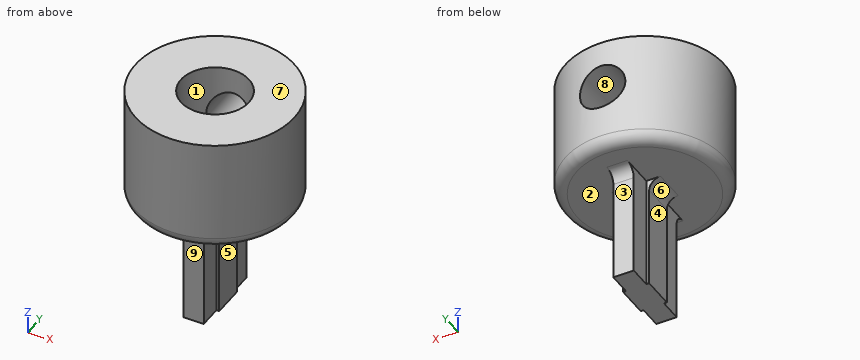
Autodesk Inventor part; units mm, degrees
ref_plane "YZ Plane" through (0, 0, 0) normal (1, 0, 0) x (0, 1, 0)
ref_plane "XZ Plane" through (0, 0, 0) normal (0, 1, 0) x (-1, 0, 0)
ref_plane "XY Plane" through (0, 0, 0) normal (0, 0, 1) x (1, 0, 0)
sketch "Sketch1" plane through (0, 0, 0) normal (0, 0, 1) x (1, 0, 0)
  line L0 (1.25, -1.5) -> (1, -1.5)
  line L1 (1, -1.5) -> (1, -3.5)
  line L2 (1, -3.5) -> (-1, -3.5)
  line L3 (-1, -3.5) -> (-1, -1.5)
  line L4 (-1, -1.5) -> (-1.25, -1.5)
  line L5 (-1.25, -1.5) -> (-1.25, 1.5)
  line L6 (-1.25, 1.5) -> (-1, 1.5)
  line L7 (-1, 1.5) -> (-1, 3.5)
  line L8 (-1, 3.5) -> (1, 3.5)
  line L9 (1, 3.5) -> (1, 1.5)
  line L10 (1, 1.5) -> (1.25, 1.5)
  line L11 (1.25, 1.5) -> (1.25, -1.5)
  circle A0 centre (4.5, 0) radius 1.55
  circle A1 centre (-4.5, 0) radius 1.55
  circle A2 centre (0, 0) radius 8
  line L12 (-0.9, -1.4) -> (-0.9, -3.4)
  line L13 (-0.9, -3.4) -> (0.9, -3.4)
  line L14 (0.9, -3.4) -> (0.9, -1.4)
  line L15 (0.9, -1.4) -> (1.15, -1.4)
  line L16 (1.15, -1.4) -> (1.15, 1.4)
  line L17 (1.15, 1.4) -> (0.9, 1.4)
  line L18 (0.9, 1.4) -> (0.9, 3.4)
  line L19 (0.9, 3.4) -> (-0.9, 3.4)
  line L20 (-0.9, 3.4) -> (-0.9, 1.4)
  line L21 (-0.9, 1.4) -> (-1.15, 1.4)
  line L22 (-1.15, 1.4) -> (-1.15, -1.4)
  line L23 (-1.15, -1.4) -> (-0.9, -1.4)
  point P0 (0, 0)
  dimension "d0" = 0.1
extrude "Extrusion1" add sketch "Sketch1" against normal blind 7 contours L23 L22 L21 L20 L19 L18 L17 L16 L15 L14 L13 L12
sketch "Sketch2" plane through (0, 0, 0) normal (0, 0, 1) x (1, 0, 0)
  line L0 (-0.9, -3.4) -> (0.9, -3.4)
  line L1 (0.9, -3.4) -> (0.9, -1.4)
  line L2 (0.9, -1.4) -> (1.15, -1.4)
  line L3 (1.15, -1.4) -> (1.15, 1.4)
  line L4 (1.15, 1.4) -> (0.9, 1.4)
  line L5 (0.9, 1.4) -> (0.9, 3.4)
  line L6 (0.9, 3.4) -> (-0.9, 3.4)
  line L7 (-0.9, 3.4) -> (-0.9, 1.4)
  line L8 (-0.9, 1.4) -> (-1.15, 1.4)
  line L9 (-1.15, 1.4) -> (-1.15, -1.4)
  line L10 (-1.15, -1.4) -> (-0.9, -1.4)
  line L11 (-0.9, -1.4) -> (-0.9, -3.4)
  point P0 (0, 0)
extrude "Extrusion2" add sketch "Sketch2" along normal blind 3
sketch "Sketch3" plane through (0, 0, 3) normal (0, 0, 1) x (1, 0, 0)
  circle A0 centre (0, 0) radius 3
  line L0 (0, 0) -> (-1.5, 0)
  line L1 (-1.5, -2.5981) -> (-1.5, 2.5981)
  line L2 (-1.5, -2.5981) -> (3.6962, -2.5981) construction
  circle A1 centre (0, 0) radius 7
  dimension "d5" = 6
  dimension "d6" = 1.5
  dimension "d7" = 90
  dimension "d8" = 14
extrude "Extrusion3" add sketch "Sketch3" along normal blind 2 contours A0 L1 | L1 A0 | A1
sketch "Sketch4" plane through (0, 0, 5) normal (0, 0, 1) x (1, 0, 0)
  circle A0 centre (0, 0) radius 3
  line L0 (0, 0) -> (0, -1.5)
  line L1 (2.5981, -1.5) -> (-2.5981, -1.5)
  circle A1 centre (0, 0) radius 7
  dimension "d11" = 6
  dimension "d12" = 1.5
extrude "Extrusion4" add sketch "Sketch4" along normal blind 10
fillet "Fillet1" radius 1 1 edges at (-7, 0, 3)
fillet "Fillet2" radius 1 4 edges at (0, -3.4, 3) (1.15, 0, 3) (-1.15, 0, 3) (0, 3.4, 3)
sketch "Sketch6" plane through (0, 0, 15) normal (0, 0, 1) x (1, 0, 0)
  circle A0 centre (0, 0) radius 5
  circle A1 centre (0, 0) radius 3
  circle A2 centre (0, 0) radius 3
  circle A3 centre (0, 0) radius 7
  point P0 (-2.5981, -1.5)
  point P1 (2.5981, -1.5)
extrude "Extrusion6" cut sketch "Sketch6" against normal blind 2 contours A0 | A1 | A3
ref_plane "Work Plane2" through (0, 7, 3) normal (0, -1, 0) x (1, 0, 0)
ref_plane "Work Plane1" through (20.4658, -7.5, 10.75) normal (0, -1, 0) x (1, 0, 0)
sketch "Sketch8" plane through (0, 7, 3) normal (0, -1, 0) x (1, 0, 0)
  circle A0 centre (0, 5.7603) radius 2
  point P0 (0, -3)
  dimension "d22" = 4
extrude "Extrusion7" cut sketch "Sketch8" along normal blind 5
properties part number "Pot_adapter"
For this review, take the finished solid that the model builds, in its own axes (mm). Face numbers are marked on the shaded views. A direction names the side the tool comes from. Give positions to 0.01 mm unless a question says otherwise; leave off trailing zeros. Write each loop counter-clockwise with the first axis right and the second up, starting at its lowest first coordinate (ties: lowest second). Pieces come first, ordered by that corner, then holes. Notation, with made-up numbers: M -19,26.5 L -2,26.5 A25 ccw -2,40.5 Z; hole C 81.25,-11 d2. An arc over 180 degrees is marked long. One line per item, written item: value.
1) Take a section at B-B, the plane y = 0. Write out the cut boundary in (x, z).
Results are:
outline: M -7,4 A1 ccw -6,3 L -2.15,3 A1 cw -1.15,2 L -1.15,-7 L 1.15,-7 L 1.15,2 A1 cw 2.15,3 L 6,3 A1 ccw 7,4 L 7,13 L 3,13 L 3,5 L -3,5 L -3,13 L -7,13 Z
2) Take a section at A-A, the plane x = 0. Write out the cut boundary in (y, z).
Results are:
outline: M -7,4 A1 ccw -6,3 L -4.4,3 A1 cw -3.4,2 L -3.4,-7 L 3.4,-7 L 3.4,2 A1 cw 4.4,3 L 6,3 A1 ccw 7,4 L 7,6.76 L 3,6.76 L 3,5 L -3,5 L -3,13 L -7,13 Z; M 3,10.76 L 7,10.76 L 7,13 L 3,13 Z
3) For the marked faces 1, 2, 3, 4 and 5, list the 3-axis set-ups (+Z, -Z, +X, -X, +Y, -Y) from which the entire face can be reached by the end or side of a thin tool; tool diameter is ignored.
Results are:
face 1: +Z
face 2: -Z
face 3: -Z, +X, -X, +Y
face 4: -Z, -X, +Y, -Y
face 5: -Z, +X, +Y, -Y
4) The part is to be moulded in two halves that separate along Z. For the marked faces 6, 7, 8 and 9, say which applies: +Z half, -Z half, draft (parallel to the pull), parting line (faces both ways), or undercut.
Results are:
face 6: -Z half
face 7: +Z half
face 8: undercut
face 9: draft
5) Take a section at C-C, the plane z = -2.75. Write out the cut boundary in (x, y).
Results are:
outline: M -1.15,-1.4 L -0.9,-1.4 L -0.9,-3.4 L 0.9,-3.4 L 0.9,-1.4 L 1.15,-1.4 L 1.15,1.4 L 0.9,1.4 L 0.9,3.4 L -0.9,3.4 L -0.9,1.4 L -1.15,1.4 Z
6) For line 1 (Y direction, x = 0, z = 11.75); line 2 (Z direction, x = 0, y = 5.65); line 3 (Y direction, x = 0, z = 8.75), list the stretches that pass through material, from the lowest coordinate up. Write a range as from..to.
Results are:
line 1: y = -7..-3, 3..7
line 2: z = 3..6.76, 10.76..13
line 3: y = -7..-3
7) For P1, Ø1, axis at x = 2, z = -4, coming from the -Y side (3 decimals); P2, Ø0.8, axis at y = 0, z = -1.5, coming from the -X side; P3, Ø4, axis at x = -3, z = 10, coming from the -Y side; P4, Ø6, axis at x = -1.5, z = 7, coming from the -Y side, all flat-tipped, find the tip position at first contact; note any pin that passes through.
Results are:
P1: passes through
P2: stops at x = -1.15
P3: stops at y = -6.93
P4: stops at y = -7
8) Take a section at D-D, the plane z = 2.75. Write out the cut boundary in (x, y).
Results are:
outline: M -1.49,-1.4 L -0.9,-1.4 L -0.9,-3.74 L 0.9,-3.74 L 0.9,-1.4 L 1.49,-1.4 L 1.49,1.4 L 0.9,1.4 L 0.9,3.74 L -0.9,3.74 L -0.9,1.4 L -1.49,1.4 Z
